from build123d import *

# Parameters (mm, degrees)
SKETCH1_R           = 5
BOSS_EXTRUDE1_DEPTH = 35
SKETCH3_R           = 10
BOSS_EXTRUDE3_DEPTH = 4
BOSS_EXTRUDE4_START = 24
SKETCH4_R           = 6
SKETCH4_R_2         = 5
BOSS_EXTRUDE4_DEPTH = 24
CUT_EXTRUDE1_DEPTH  = 42.484937025
FILLET1_R           = 1
SKETCH6_R           = 3.5
CUT_EXTRUDE2_DEPTH  = 24
CHAMFER1_SIZE       = 2
FILLET2_R           = 10
SKETCH7_R           = 1.5
BOSS_EXTRUDE5_DEPTH = 8
FILLET3_R           = 4
CUT_REVOLVE1_ANGLE  = 200
SKETCH9_R           = 1.8
SKETCH9_R_2         = 1.5
BOSS_EXTRUDE6_DEPTH = 3
SKETCH10_R          = 3.5
BOSS_EXTRUDE7_DEPTH = 10
SKETCH14_W          = 13
SKETCH14_H          = 12
CUT_EXTRUDE3_DEPTH  = 4
FILLET4_R           = 2


with BuildPart() as part:
    # Sketch1 → Boss-Extrude1 (new body)
    with BuildSketch(Plane.XY):
        Circle(SKETCH1_R)
    extrude(amount=BOSS_EXTRUDE1_DEPTH)

    # Sketch3 → Boss-Extrude3 (add)
    with BuildSketch(Plane.XY.offset(35)):
        Circle(SKETCH3_R)
    extrude(amount=BOSS_EXTRUDE3_DEPTH)

    # Sketch4 → Boss-Extrude4 (add)
    with BuildSketch(Plane(origin=(0, 0, 35), x_dir=(-1, 0, 0), z_dir=(0, 0, -1)).offset(BOSS_EXTRUDE4_START)):
        with Locations(Location((0, 0, 0), (0, 0, 180))):
            Circle(SKETCH4_R)
        Circle(SKETCH4_R_2, mode=Mode.SUBTRACT)
    extrude(amount=-BOSS_EXTRUDE4_DEPTH)

    # Sketch5 → Cut-Extrude1 (cut, through all)
    with BuildSketch(Plane.XY.offset(39)):
        with BuildLine():
            ThreePointArc((-1.8, 9.836666102), (-6.99867823, 7.142723782), (-9.797958971, 2))
            Line((-9.797958971, 2), (-6, 2))
            Line((-6, 2), (-1.8, 9.836666102))
        make_face()
        with BuildLine():
            ThreePointArc((9.797958971, 2), (6.99867823, 7.142723782), (1.8, 9.836666102))
            Line((1.8, 9.836666102), (6, 2))
            Line((6, 2), (9.797958971, 2))
        make_face()
    extrude(amount=-CUT_EXTRUDE1_DEPTH, mode=Mode.SUBTRACT)

    # Fillet1
    fillet1_edges = [part.edges().sort_by_distance(p)[0] for p in [
        (-9.797958971, 2, 37),
        (-1.8, 9.836666102, 37),
        (1.8, 9.836666102, 37),
        (9.797958971, 2, 37),
    ]]
    fillet(fillet1_edges, radius=FILLET1_R)

    # Sketch6 → Cut-Extrude2 (cut)
    with BuildSketch(Plane.XY.offset(39)):
        Circle(SKETCH6_R)
    extrude(amount=-CUT_EXTRUDE2_DEPTH, mode=Mode.SUBTRACT)

    # Chamfer1
    chamfer1_edges = [part.edges().sort_by_distance(p)[0] for p in [
        (-3.5, 0, 39),
    ]]
    chamfer(chamfer1_edges, length=CHAMFER1_SIZE)

    # Fillet2
    # the kernel refuses this fillet: 10 mm, written as the material it takes off along each edge
    with BuildSketch(Plane(origin=(0, 0, 37), x_dir=(1, 0, 0), z_dir=(0, -1, 0))) as fillet2_piece_1:
        with BuildLine():
            CenterArc((13.5, -4), FILLET2_R, 143.130102354, 36.869897646)
            Line((3.5, -4), (3.3, -4))
            Line((3.3, -4), (3.3, 0))
            Line((3.3, 0), (3.358578644, 0.141421356))
            ThreePointArc((3.358578644, 0.141421356), (4.358578644, 1.141421356), (5.34, 2.12))
            Line((5.34, 2.12), (5.5, 2))
        make_face()
    revolve(axis=Axis((0, 0, 37), (0, 0, 1)), mode=Mode.SUBTRACT)

    # Sketch7 → Boss-Extrude5 (add)
    with BuildSketch(Plane.XY.offset(39)):
        with Locations((0, 8)):
            Circle(SKETCH7_R)
    extrude(amount=BOSS_EXTRUDE5_DEPTH)

    # Fillet3
    fillet3_edges = [part.edges().sort_by_distance(p)[0] for p in [
        (-6, 2, 37),
        (6, 2, 37),
    ]]
    fillet(fillet3_edges, radius=FILLET3_R)

    # Sketch8 → Cut-Revolve1 (revolve, symmetric, cut)
    with BuildSketch(Plane(origin=(0, 0, 0), x_dir=(0, 0, -1), z_dir=(1, 0, 0))) as cut_revolve1_sk:
        Polygon((-38.217890117, -9.976578367), (-39, -8.976578367), (-39, -9.976578367), align=None)
    revolve(axis=Axis((0, 0, 1000), (0, 0, -1)), revolution_arc=CUT_REVOLVE1_ANGLE / 2, mode=Mode.SUBTRACT)
    revolve(cut_revolve1_sk.sketch, axis=Axis((0, 0, 1000), (0, 0, 1)), revolution_arc=CUT_REVOLVE1_ANGLE / 2, mode=Mode.SUBTRACT)

    # Sketch9 → Boss-Extrude6 (add)
    with BuildSketch(Plane.XY.offset(39)):
        with Locations((0, 8)):
            Circle(SKETCH9_R)
        with Locations((0, 8)):
            Circle(SKETCH9_R_2, mode=Mode.SUBTRACT)
    extrude(amount=BOSS_EXTRUDE6_DEPTH)

    # Sketch10 → Boss-Extrude7 (add)
    with BuildSketch(Plane(origin=(0, 0, 0), x_dir=(-1, 0, 0), z_dir=(0, 0, -1))):
        with Locations(Location((0, 0, 0), (0, 0, 180))):
            Circle(SKETCH10_R)
    extrude(amount=BOSS_EXTRUDE7_DEPTH)

    # Sketch14 → Cut-Extrude3 (cut)
    with BuildSketch(Plane(origin=(5.977168189, -0.522934456, 0), x_dir=(0, 0, -1), z_dir=(0.9961946980917453, -0.08715574274766187, 0))):
        with Locations((-22.5, 0)):
            Rectangle(SKETCH14_W, SKETCH14_H)
    extrude(amount=-CUT_EXTRUDE3_DEPTH, mode=Mode.SUBTRACT)

    # Fillet4
    # the kernel refuses this fillet: 2 mm, written as the material it adds along each edge
    with BuildSketch(Plane(origin=(1.806946495, -2.29393355, 16), x_dir=(0, 0, 1), z_dir=(0.08715574274766187, 0.9961946980917453, 0))) as fillet4_piece_1_section:
        with BuildLine():
            CenterArc((FILLET4_R, FILLET4_R), FILLET4_R, 180, 90)
            Line((0, FILLET4_R), (0, 0))
            Line((0, 0), (FILLET4_R, 0))
        make_face()
    fillet4_piece_1 = extrude(amount=12.784572926, mode=Mode.PRIVATE)
    fillet4_piece_1 = fillet4_piece_1 - Plane(origin=(0, 0, 16.407191897), x_dir=(1, 0, 0), z_dir=(0, 0, 1)) * Cylinder(3.5, 34, mode=Mode.PRIVATE)
    fillet4_piece_1 = fillet4_piece_1 & Plane(origin=(0, 0, 16.407191897), x_dir=(1, 0, 0), z_dir=(0, 0, -1)) * Cylinder(6, 34, mode=Mode.PRIVATE)
    add(fillet4_piece_1)
    with BuildSketch(Plane(origin=(1.063583349, -10.790613187, 16), x_dir=(0.9961946980917453, -0.08715574274766187, 0), z_dir=(0.08715574274766187, 0.9961946980917453, 0))) as fillet4_piece_2_section:
        with BuildLine():
            CenterArc((FILLET4_R, -FILLET4_R), FILLET4_R, 90, 90)
            Line((0, -FILLET4_R), (0, 0))
            Line((0, 0), (FILLET4_R, 0))
        make_face()
    fillet4_piece_2 = extrude(amount=12.784572926, mode=Mode.PRIVATE)
    fillet4_piece_2 = fillet4_piece_2 - Plane(origin=(0, 0, 16.407193431), x_dir=(1, 0, 0), z_dir=(0, 0, 1)) * Cylinder(3.5, 34, mode=Mode.PRIVATE)
    fillet4_piece_2 = fillet4_piece_2 & Plane(origin=(0, 0, 16.407193431), x_dir=(1, 0, 0), z_dir=(0, 0, -1)) * Cylinder(6, 34, mode=Mode.PRIVATE)
    add(fillet4_piece_2)
    with BuildSketch(Plane(origin=(2.177832298, 1.945310579, 29), x_dir=(0, 0, -1), z_dir=(-0.08715574274766187, -0.9961946980917453, 0))) as fillet4_piece_3_section:
        with BuildLine():
            CenterArc((FILLET4_R, FILLET4_R), FILLET4_R, 180, 90)
            Line((0, FILLET4_R), (0, 0))
            Line((0, 0), (FILLET4_R, 0))
        make_face()
    fillet4_piece_3 = extrude(amount=12.784572926, mode=Mode.PRIVATE)
    fillet4_piece_3 = fillet4_piece_3 - Plane(origin=(0, 0, 28.592806917), x_dir=(1, 0, 0), z_dir=(0, 0, 1)) * Cylinder(3.5, 34, mode=Mode.PRIVATE)
    fillet4_piece_3 = fillet4_piece_3 & Plane(origin=(0, 0, 28.592806917), x_dir=(1, 0, 0), z_dir=(0, 0, -1)) * Cylinder(6, 34, mode=Mode.PRIVATE)
    add(fillet4_piece_3)
    with BuildSketch(Plane(origin=(2.921195444, 10.441990216, 29), x_dir=(0, 0, -1), z_dir=(-0.08715574274766187, -0.9961946980917453, 0))) as fillet4_piece_4_section:
        with BuildLine():
            CenterArc((FILLET4_R, FILLET4_R), FILLET4_R, 180, 90)
            Line((0, FILLET4_R), (0, 0))
            Line((0, 0), (FILLET4_R, 0))
        make_face()
    fillet4_piece_4 = extrude(amount=12.784572926, mode=Mode.PRIVATE)
    fillet4_piece_4 = fillet4_piece_4 - Plane(origin=(0, 0, 28.592808103), x_dir=(1, 0, 0), z_dir=(0, 0, 1)) * Cylinder(3.5, 34, mode=Mode.PRIVATE)
    fillet4_piece_4 = fillet4_piece_4 & Plane(origin=(0, 0, 28.592808103), x_dir=(1, 0, 0), z_dir=(0, 0, -1)) * Cylinder(6, 34, mode=Mode.PRIVATE)
    add(fillet4_piece_4)


solid = part.part
Can you work these out from the model? Positions are in its coordinate system, mm. A direction names the side the tool comes from. Round coordinates to 2 decimals unless told otherwise and drop trailing zeros. Order: outer loops, then holes, each group sorted by start corner. A loop starts at its lowest first (then second) coordinate and runs counter-clockwise, first axis right, second up. Notation, with made-up numbers: M -32,65 L 22,65 A7 ccw 22,73 Z; hole C 87.5,-24.5 d1. An arc over 180 degrees is marked long. Use a Markdown table: item, result.
1) Imagine slicing it at D-D (z = 43). List the corners of the cut face in (x, y) for me, then the cut area to 3 significant figures.
Geometry says:
| item | result |
|---|---|
| outline | C 0,8 d3 |
| area | 7.07 mm² |
2) On a 3-axis mill with a long thin cutter (end or side, diameter ignored), from which of +Z, -Z, +X, -X, +Y, -Y can I reach the whole of each face in a straight line? I mean faces 1 (the face through (3.84, -0.256, 28.994)), 2 (the face through (-1.08, -4.88, 5.42)), 3 (the face through (9.603, 1.752, 36.972)). Say none if no direction works.
Geometry says:
| item | result |
|---|---|
| face 1 | +X, -Y |
| face 2 | -Z |
| face 3 | +Z, -Z, +X, +Y |
3) If we mould it in two halves opening along Z, with no side actions, what happens to faces 4 (the face through (1.622, -4.403, 22.563)), 5 (the face through (0, 8, 47)), 6 (the face through (3.432, 6.791, 37.028))? For each: +Z half, -Z half, draft (parallel to the pull), parting line (faces both ways), or undercut.
Geometry says:
| item | result |
|---|---|
| face 4 | undercut |
| face 5 | +Z half |
| face 6 | draft |
4) Imagine slicing it at B-B (y = 8). List the corners of the cut face in (x, z) for me.
Geometry says:
| item | result |
|---|---|
| outline | M -2.78,35 L 2.78,35 L 2.78,39 L 1.8,39 L 1.8,42 L 1.5,42 L 1.5,47 L -1.5,47 L -1.5,42 L -1.8,42 L -1.8,39 L -2.78,39 Z |
5) If I drill on line 1 along Z through (x, y) = (-8, -3.25); line 2 along Z through (x, y) = (3, 0.25); line 3 along X through (y, z) = (-0.5, -6.5), over which ranges is the centre line in solid material (lowest first)?
Geometry says:
| item | result |
|---|---|
| line 1 | z = 35 to 39 |
| line 2 | z = -10 to 15 |
| line 3 | x = -3.46 to 3.46 |
6) Imagine slicing it at C-C (z = 3). List the corners of the cut face in (x, y) for me, then the cut area to 3 significant figures.
Geometry says:
| item | result |
|---|---|
| outline | C 0,0 d10 |
| area | 78.5 mm² |
7) I'm going to push flat-ended pins straight in: P1, Ø8, axis at x = 7.5, z = 35, coming from the +Y side; P2, Ø0.7, axis at x = 5, y = 1.5, coming from the +Z side; P3, Ø0.7, axis at x = 5, y = -2, coming from the -Z side. Where does each tip first touch, or does it pass through?
Geometry says:
| item | result |
|---|---|
| P1 | stops at y = 6.66 |
| P2 | stops at z = 39 |
| P3 | stops at z = 11 |
